Geometry: final body of the model. Coordinates: model frame, mm. Give positions to 0.01 mm unless a question says otherwise; leave off trailing zeros. Order: outer loops, then holes, each group sorted by start corner. A loop starts at its lowest first (then second) coordinate and runs counter-clockwise, first axis right, second up. Notation, with made-up numbers: (24, -11) -> (73, -11) arc R19 cw to (73, 8) -> close; hole circle Ø8 at (29, 73.25). An arc over 180 degrees is marked (long way). One line per question, with ' | ' between items. Start each with the question number.
(1) Ray query, L1, parallel to X at y = 31.5, z = -26; L2, parallel to X at y = 31.5, z = -80.5; L3, parallel to Y at x = 3.75, z = -45.5. Return the intervals inside material, ascending.
(2) First-contact query: pin 1 Ø2.5 at (x, z) = (-11.92, 0.25) entering from -Y; pin 2 Ø12 at (y, z) = (22, -76.5) entering from -X; pin 3 Ø0.9 at (x, z) = (12, 0) entering from +Y; pin 4 Ø1.5 at (y, z) = (24, -23.5) entering from -X. Flat tips, straight axial feed; report the tip coordinate or a pass-through.
(3) Section B-B (y = 24). Return loops of the section in (x, z), then the cut area to 3 significant figures.
(4) Section A-A (z = -42.5). Return loops of the section in (x, y).
```python
from build123d import *

# Parameters (mm, degrees)
BOSS_EXTRUDE1_DEPTH            = 35
SKETCH2_R                      = 2.6
SKETCH2_R_2                    = 1.55
BOSS_EXTRUDE3_DEPTH            = 5
CUT_EXTRUDE1_REACH             = 101.661
CUT_EXTRUDE1_DIRECTION_2_DEPTH = 100.661000569
CUT_EXTRUDE2_REACH             = 101.661
CUT_EXTRUDE2_DIRECTION_2_DEPTH = 100.661000569
FILLET1_R                      = 2
SKETCH6_R                      = 2.6
BOSS_EXTRUDE4_DEPTH            = 1


with BuildPart() as part:
    # Sketch1 → Boss-Extrude1 (new body)
    with BuildSketch(Plane(origin=(0, 0, 0), x_dir=(1, 0, 0), z_dir=(0, 1, 0))):
        Polygon((-13.5, 0), (0, 83.718518379), (13.5, 0), (14.487246657, 0.15919811), (0, 90), (-14.487246657, 0.15919811), align=None)
    extrude(amount=BOSS_EXTRUDE1_DEPTH)

    # Sketch2 → Boss-Extrude3 (add)
    # profile 1 of 8: a face of its own
    with BuildSketch(Plane(origin=(0, 0, 0), x_dir=(1, 0, 0), z_dir=(0, 1, 0))):
        with Locations((11.920405349, -0.254716975)):
            Circle(SKETCH2_R)
        with Locations(Location((11.920405349, -0.254716975, 0), (0, 0, 270))):
            Circle(SKETCH2_R_2, mode=Mode.SUBTRACT)
    # profile 2 of 8: a face of its own
    with BuildSketch(Plane(origin=(0, 0, 0), x_dir=(1, 0, 0), z_dir=(0, 1, 0))):
        with Locations((9.373235594, 15.541229537)):
            Circle(SKETCH2_R)
        with Locations(Location((9.373235594, 15.541229537, 0), (0, 0, 270))):
            Circle(SKETCH2_R_2, mode=Mode.SUBTRACT)
    # profile 3 of 8: a face of its own
    with BuildSketch(Plane(origin=(0, 0, 0), x_dir=(1, 0, 0), z_dir=(0, 1, 0))):
        with Locations((6.826065839, 31.33717605)):
            Circle(SKETCH2_R)
        with Locations(Location((6.826065839, 31.33717605, 0), (0, 0, 270))):
            Circle(SKETCH2_R_2, mode=Mode.SUBTRACT)
    # profile 4 of 8: a face of its own
    with BuildSketch(Plane(origin=(0, 0, 0), x_dir=(1, 0, 0), z_dir=(0, 1, 0))):
        with Locations((4.278896085, 47.133122563)):
            Circle(SKETCH2_R)
        with Locations(Location((4.278896085, 47.133122563, 0), (0, 0, 270))):
            Circle(SKETCH2_R_2, mode=Mode.SUBTRACT)
    # profile 5 of 8: a face of its own
    with BuildSketch(Plane(origin=(0, 0, 0), x_dir=(1, 0, 0), z_dir=(0, 1, 0))):
        with Locations((-4.278896085, 47.133122563)):
            Circle(SKETCH2_R)
        with Locations(Location((-4.278896085, 47.133122563, 0), (0, 0, 90))):
            Circle(SKETCH2_R_2, mode=Mode.SUBTRACT)
    # profile 6 of 8: a face of its own
    with BuildSketch(Plane(origin=(0, 0, 0), x_dir=(1, 0, 0), z_dir=(0, 1, 0))):
        with Locations((-6.826065839, 31.33717605)):
            Circle(SKETCH2_R)
        with Locations(Location((-6.826065839, 31.33717605, 0), (0, 0, 90))):
            Circle(SKETCH2_R_2, mode=Mode.SUBTRACT)
    # profile 7 of 8: a face of its own
    with BuildSketch(Plane(origin=(0, 0, 0), x_dir=(1, 0, 0), z_dir=(0, 1, 0))):
        with Locations((-9.373235594, 15.541229537)):
            Circle(SKETCH2_R)
        with Locations(Location((-9.373235594, 15.541229537, 0), (0, 0, 90))):
            Circle(SKETCH2_R_2, mode=Mode.SUBTRACT)
    # profile 8 of 8: a face of its own
    with BuildSketch(Plane(origin=(0, 0, 0), x_dir=(1, 0, 0), z_dir=(0, 1, 0))):
        with Locations((-11.920405349, -0.254716975)):
            Circle(SKETCH2_R)
        with Locations(Location((-11.920405349, -0.254716975, 0), (0, 0, 90))):
            Circle(SKETCH2_R_2, mode=Mode.SUBTRACT)
    boss_extrude3 = extrude(amount=BOSS_EXTRUDE3_DEPTH)

    # Cut-Extrude1: up to this face of the body (flat: up to its plane)
    cut_extrude1_end = Plane(part.part.faces().sort_by_distance((-6.691549619, 17.871487916, -42.221731728))[0])
    # Sketch4 → Cut-Extrude1 (cut, up to the picked face)
    with BuildSketch(Plane(origin=(0.342144515, 0, 2.121765321), x_dir=(0.9872466570606503, 0, -0.1591981096702188), z_dir=(0.1591981096702188, 0, 0.9872466570606503)), mode=Mode.PRIVATE) as cut_extrude1_sk1:
        Polygon((13.32782987, 5), (9.12782987, 5), (9.12782987, 1.475781549), align=None)
    cut_extrude1_tool1 = split(extrude(cut_extrude1_sk1.sketch, amount=-CUT_EXTRUDE1_REACH, mode=Mode.PRIVATE), bisect_by=cut_extrude1_end, keep=Keep.BOTH, mode=Mode.PRIVATE)
    cut_extrude1 = cut_extrude1_tool1.solids().sort_by(Axis((10.735709, 3.825261, 0.445755), (-0.1591981096702188, 0, -0.9872466570606503)))[0]
    add(cut_extrude1, mode=Mode.SUBTRACT)

    # Sketch4 → Cut-Extrude1 direction 2 (cut)
    with BuildSketch(Plane(origin=(0.342144515, 0, 2.121765321), x_dir=(0.9872466570606503, 0, -0.1591981096702188), z_dir=(0.1591981096702188, 0, 0.9872466570606503))):
        Polygon((13.32782987, 5), (9.12782987, 5), (9.12782987, 1.475781549), align=None)
    cut_extrude1_direction_2 = extrude(amount=CUT_EXTRUDE1_DIRECTION_2_DEPTH, mode=Mode.SUBTRACT)

    # Cut-Extrude2: up to this face of the body (flat: up to its plane)
    cut_extrude2_end = Plane(part.part.faces().sort_by_distance((6.691549619, 17.871487916, -42.221731728))[0])
    # Sketch5 → Cut-Extrude2 (cut, up to the picked face)
    with BuildSketch(Plane(origin=(-0.342144515, 0, 2.121765321), x_dir=(0.9872466570606502, 0, 0.15919810967021986), z_dir=(-0.15919810967021986, 0, 0.9872466570606502)), mode=Mode.PRIVATE) as cut_extrude2_sk1:
        Polygon((-9.12782987, 5), (-9.12782987, 1.475781549), (-13.32782987, 5), align=None)
    cut_extrude2_tool1 = split(extrude(cut_extrude2_sk1.sketch, amount=-CUT_EXTRUDE2_REACH, mode=Mode.PRIVATE), bisect_by=cut_extrude2_end, keep=Keep.BOTH, mode=Mode.PRIVATE)
    cut_extrude2 = cut_extrude2_tool1.solids().sort_by(Axis((-10.735709, 3.825261, 0.445755), (0.15919810967021986, 0, -0.9872466570606502)))[0]
    add(cut_extrude2, mode=Mode.SUBTRACT)

    # Sketch5 → Cut-Extrude2 direction 2 (cut)
    with BuildSketch(Plane(origin=(-0.342144515, 0, 2.121765321), x_dir=(0.9872466570606502, 0, 0.15919810967021986), z_dir=(-0.15919810967021986, 0, 0.9872466570606502))):
        Polygon((-9.12782987, 5), (-9.12782987, 1.475781549), (-13.32782987, 5), align=None)
    cut_extrude2_direction_2 = extrude(amount=CUT_EXTRUDE2_DIRECTION_2_DEPTH, mode=Mode.SUBTRACT)

    # Mirror2: Boss-Extrude3, Cut-Extrude1, Cut-Extrude1 direction 2, Cut-Extrude2, Cut-Extrude2 direction 2 across plane
    add(boss_extrude3.mirror(Plane.ZX.offset(17.5)))
    add(cut_extrude1.mirror(Plane.ZX.offset(17.5)), mode=Mode.SUBTRACT)
    add(cut_extrude1_direction_2.mirror(Plane.ZX.offset(17.5)), mode=Mode.SUBTRACT)
    add(cut_extrude2.mirror(Plane.ZX.offset(17.5)), mode=Mode.SUBTRACT)
    add(cut_extrude2_direction_2.mirror(Plane.ZX.offset(17.5)), mode=Mode.SUBTRACT)

    # Fillet1
    # the kernel refuses this fillet: 2 mm, written as the material it adds along each edge
    with BuildSketch(Plane(origin=(-19.423479942, 5, -0.955188658), x_dir=(-0.15919810967021975, 0, 0.9872466570606501), z_dir=(0.9872466570606501, 0, 0.15919810967021975))) as fillet1_piece_1_section:
        with BuildLine():
            CenterArc((FILLET1_R, -FILLET1_R), FILLET1_R, 90, 90)
            Line((0, -FILLET1_R), (0, 0))
            Line((0, 0), (FILLET1_R, 0))
        make_face()
    fillet1_piece_1 = extrude(amount=6, mode=Mode.PRIVATE)
    fillet1_piece_1 = fillet1_piece_1 & Plane(origin=(-11.920405349, 5.222362792, 0.254716975), x_dir=(1, 0, 0), z_dir=(0, -1, 0)) * Cylinder(2.6, 21, mode=Mode.PRIVATE)
    add(fillet1_piece_1)
    with BuildSketch(Plane(origin=(13.5, 5, 0), x_dir=(0, 1, 0), z_dir=(0.9872466570606502, 0, -0.15919810967021866))) as fillet1_piece_2_section:
        with BuildLine():
            CenterArc((FILLET1_R, FILLET1_R), FILLET1_R, 180, 90)
            Line((0, FILLET1_R), (0, 0))
            Line((0, 0), (FILLET1_R, 0))
        make_face()
    fillet1_piece_2 = extrude(amount=6, mode=Mode.PRIVATE)
    fillet1_piece_2 = fillet1_piece_2 & Plane(origin=(11.920405349, 5.699977741, 0.254716975), x_dir=(1, 0, 0), z_dir=(0, -1, 0)) * Cylinder(2.6, 20, mode=Mode.PRIVATE)
    add(fillet1_piece_2)
    with BuildSketch(Plane(origin=(13.5, 30, 0), x_dir=(0, -1, 0), z_dir=(0.9872466570606502, 0, -0.15919810967021866))) as fillet1_piece_3_section:
        with BuildLine():
            CenterArc((FILLET1_R, -FILLET1_R), FILLET1_R, 90, 90)
            Line((0, -FILLET1_R), (0, 0))
            Line((0, 0), (FILLET1_R, 0))
        make_face()
    fillet1_piece_3 = extrude(amount=6, mode=Mode.PRIVATE)
    fillet1_piece_3 = fillet1_piece_3 & Plane(origin=(11.920405349, 29.300022259, 0.254716975), x_dir=(1, 0, 0), z_dir=(0, 1, 0)) * Cylinder(2.6, 20, mode=Mode.PRIVATE)
    add(fillet1_piece_3)
    with BuildSketch(Plane(origin=(-19.423479942, 30, -0.955188658), x_dir=(0, -1, 0), z_dir=(0.9872466570606501, 0, 0.15919810967021975))) as fillet1_piece_4_section:
        with BuildLine():
            CenterArc((FILLET1_R, -FILLET1_R), FILLET1_R, 90, 90)
            Line((0, -FILLET1_R), (0, 0))
            Line((0, 0), (FILLET1_R, 0))
        make_face()
    fillet1_piece_4 = extrude(amount=6, mode=Mode.PRIVATE)
    fillet1_piece_4 = fillet1_piece_4 & Plane(origin=(-11.920405349, 29.777637105, 0.254716975), x_dir=(1, 0, 0), z_dir=(0, 1, 0)) * Cylinder(2.6, 21, mode=Mode.PRIVATE)
    add(fillet1_piece_4)

    # Sketch6 → Boss-Extrude4 (add)
    with BuildSketch(Plane.XZ):
        with Locations((11.920405349, 0.254716975)):
            Circle(SKETCH6_R)
        with Locations((9.373235594, -15.541229537)):
            Circle(SKETCH6_R)
        with Locations((6.826065839, -31.33717605)):
            Circle(SKETCH6_R)
        with Locations((4.278896085, -47.133122563)):
            Circle(SKETCH6_R)
        with Locations((-4.278896085, -47.133122563)):
            Circle(SKETCH6_R)
        with Locations((-6.826065839, -31.33717605)):
            Circle(SKETCH6_R)
        with Locations((-9.373235594, -15.541229537)):
            Circle(SKETCH6_R)
        with Locations((-11.920405349, 0.254716975)):
            Circle(SKETCH6_R)
    extrude(amount=-BOSS_EXTRUDE4_DEPTH)


solid = part.part
```
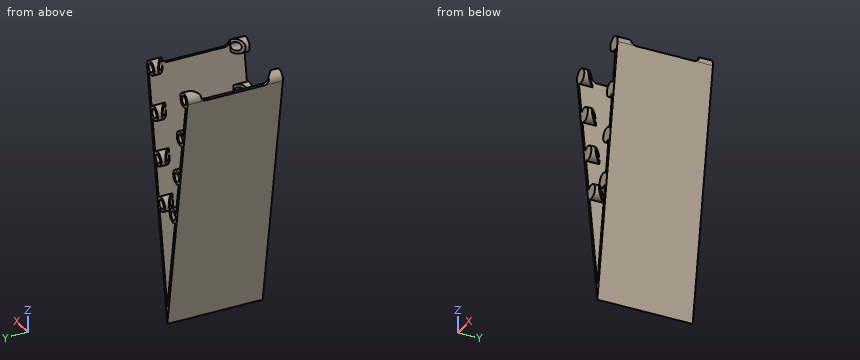
Response:
1) L1: x = -10.32 to -9.31, 9.31 to 10.32 | L2: x = -1.53 to -0.52, 0.52 to 1.53 | L3: y = 0 to 3, 32 to 35
2) pin 1: stops at y = 0 | pin 2: stops at x = -3.14 | pin 3: stops at y = 1 | pin 4: stops at x = -10.84
3) outline: (-14.49, -0.16) -> (0, -90) -> (14.49, -0.16) -> (13.5, 0) -> (0, -83.72) -> (-13.5, 0) -> close | area: 176 mm^2
4) outline: (-7.66, 0) -> (-6.65, 0) -> (-6.65, 35) -> (-7.66, 35) -> close; (6.65, 0) -> (7.66, 0) -> (7.66, 35) -> (6.65, 35) -> close
